```python
from build123d import *

# Parameters (mm, degrees)
F2_SIZE  = 3.175
F4_DEPTH = 25.4
F5_R     = 1.016
F6_R     = 1.27


with BuildPart() as f1:
    # F0 (on Front) → F1 (revolve)
    with BuildSketch(Plane.XZ):
        Polygon((-19.05, -12.7), (-5.4229, -12.7), (-5.4229, 15.875), (-7.0104, 15.875), (-7.0104, 14.2875), (-6.5024, 14.2875), (-6.5024, 12.7), (-7.0104, 12.7), (-7.0104, 6.35), (-9.779, 6.35), (-9.779, 12.7), (-13.208, 10.16), (-13.208, 6.35), (-13.208, 3.175), (-12.7, 3.175), (-12.7, 0), (-19.05, 0), (-19.05, -1.5875), (-15.875, -1.5875), (-15.875, -4.7625), (-19.05, -4.7625), align=None)
    revolve(axis=Axis((0, 0, 5.660842), (0, 0, -1)))

    # F2
    f2_edges = [f1.edges().sort_by_distance(p)[0] for p in [
        (19.05, 0, -12.7),
    ]]
    chamfer(f2_edges, length=F2_SIZE)

    # F3 (on Front) → F4 (cut)
    with BuildSketch(Plane.XZ):
        with BuildLine():
            ThreePointArc((1.5875, -4.7625), (3.175, -3.175), (1.5875, -1.5875))
            Line((1.5875, -1.5875), (-1.5875, -1.5875))
            ThreePointArc((-1.5875, -1.5875), (-3.175, -3.175), (-1.5875, -4.7625))
            Line((-1.5875, -4.7625), (1.5875, -4.7625))
        make_face()
    extrude(amount=F4_DEPTH, mode=Mode.SUBTRACT)

    # F5
    f5_edges = [f1.edges().sort_by_distance(p)[0] for p in [
        (19.05, 0, -1.5875),
        (19.05, 0, -4.7625),
    ]]
    fillet(f5_edges, radius=F5_R)

    # F6
    f6_edges = [f1.edges().sort_by_distance(p)[0] for p in [
        (5.4229, 0, 15.875),
    ]]
    fillet(f6_edges, radius=F6_R)


solid = f1.part
```
The model under review builds one solid part; all positions refer to its coordinate system, in mm. A direction names the side the tool comes from. Round coordinates to 2 decimals unless told otherwise and drop trailing zeros. Loops run counter-clockwise (first coordinate to the right, second up) from the corner with the lowest first, then second, coordinate; pieces in that order, holes last.
1) Consider section C-C on z = 2. State the section outline as (x, y) points.
Values follow:
outline: circle Ø25.4 at (0, 0); hole circle Ø10.85 at (0, 0)
2) Consider section B-B on z = -6.75. State the section outline as (x, y) points.
Values follow:
outline: circle Ø38.1 at (0, 0); hole circle Ø10.85 at (0, 0)
3) Wall thickness on line 1 along Y through (x, z) = (0, 9.5); line 2 along Y through (x, z) = (3, 6.5); line 3 along Z through (x, y) = (13.5, 3.5): over which ranges is each line inside the solid? List them lowest first.
Values follow:
line 1: y = -13.21 to -9.78, -7.01 to -5.42, 5.42 to 7.01, 9.78 to 13.21
line 2: y = -12.86 to -9.31, -6.34 to -4.52, 4.52 to 6.34, 9.31 to 12.86
line 3: z = -12.7 to 0
4) Consider section A-A on x = 0. Give the number of separate pieces and of enclosed holes in the cut face, then the cut area to 3 significant figures.
Values follow:
separate pieces: 3
enclosed holes: 0
area: 440 mm2
5) The part is to be moulded in two halves that separate along Z. For faces 6 (the face through (2.12, -9.546, 9.569)), 7 (the face through (-0.68, 15.86, -3.2)), 8 (the face through (2.17, -9.76, 12.54)), 9 (the face through (0.846, 6.447, 13.483)), say which applies: pulls with the +Z half, pulls with the -Z half, needs draft (parallel to the pull), parting line crosses it, or undercut.
Values follow:
face 6: needs draft
face 7: undercut
face 8: pulls with the +Z half
face 9: undercut
6) Tool access review of faces 1 (the face through (2.75, -12.4, 1.57)), 2 (the face through (-6.687, 2.106, 15.07)), 3 (the face through (3.175, -10.016, -3.21)), 4 (the face through (-7, 0, -12.7)), 5 (the face through (15.12, -11.59, -7.68)): name each direction out of +Z, -Z, +X, -X, +Y, -Y from which nothing blocks a thin tool from reaching the whole face with its end or side.
Values follow:
face 1: none
face 2: +Z
face 3: -Y
face 4: -Z, +X, -X, +Y, -Y
face 5: +Z, -Z
7) Consider section D-D on z = -2.75. State the section outline as (x, y) points (3 decimals).
Values follow:
outline: (-3.117, -15.566) - (-3.117, -4.438) arc R5.423 cw (long way) to (3.117, -4.438) - (3.117, -15.566) arc R15.875 ccw (long way) to start
8) Clearance check with flat-ended pins moving along their axes: P1, Ø6, axis at y = -4.5, z = 9.5, coming from the -X side; P2, Ø6, axis at x = 1.5, z = 6.5, coming from the +Y side; P3, Ø7, axis at x = -2, y = -1, coming from the +Z side; P4, Ø2, axis at x = 5.5, y = -3.5, coming from the +Z side (3 decimals). State where each tip first meets the part, or that it passes through.
Values follow:
P1: stops at x = -13.12
P2: stops at y = 13.21
P3: stops at z = 15.44
P4: stops at z = 15.875
